Input: dimensioned drawing with shaded views. Units: mm. Origin: part minimum x, y, z. A direction names the side the tool comes from. Round coordinates to 2 decimals unless told otherwise and drop trailing zeros. Loops run counter-clockwise (first coordinate to the right, second up) from the corner with the lowest first, then second, coordinate; pieces in that order, holes last.
Item 1: Pull-direction query (Z, two-part tool) for the marked faces 3, 4 and 5; classes: released by +Z, released by -Z, zero draft, split by the parting line, or undercut.
Item 2: First-contact query: P1, Ø1, axis at y = 2.5, z = 9.5, coming from the -X side; P2, Ø5, axis at x = 5.75, z = 6.75, coming from the -Y side. Flat tips, straight axial feed; report the tip coordinate or a pass-through.
Item 3: Section query B-B on z = 6.75. Return loops of the section in (x, y).
Item 4: Ray query, L1, parallel to X at y = 5.65, z = 6.75; L2, parallel to Z at x = 5.75, y = 5.3; L3, parallel to X at y = 1, z = 7. Return the intervals inside material, ascending.
Item 5: Access query for the marked faces 1 and 2. Directions: +Z, -Z, +X, -X, +Y, -Y. A direction counts if a zero-diameter tool reaches every point of the face in a straight line with its end or side. Return the directions, or none.
Item 6: Section query A-A on x = 5.75. Return loops of the section in (y, z).
Item 7: Section query D-D on z = 4. Return loops of the section in (x, y), then the cut area to 4 significant figures.
Item 8: Section query C-C on y = 6. Return loops of the section in (x, z), then the cut area to 3 significant figures.
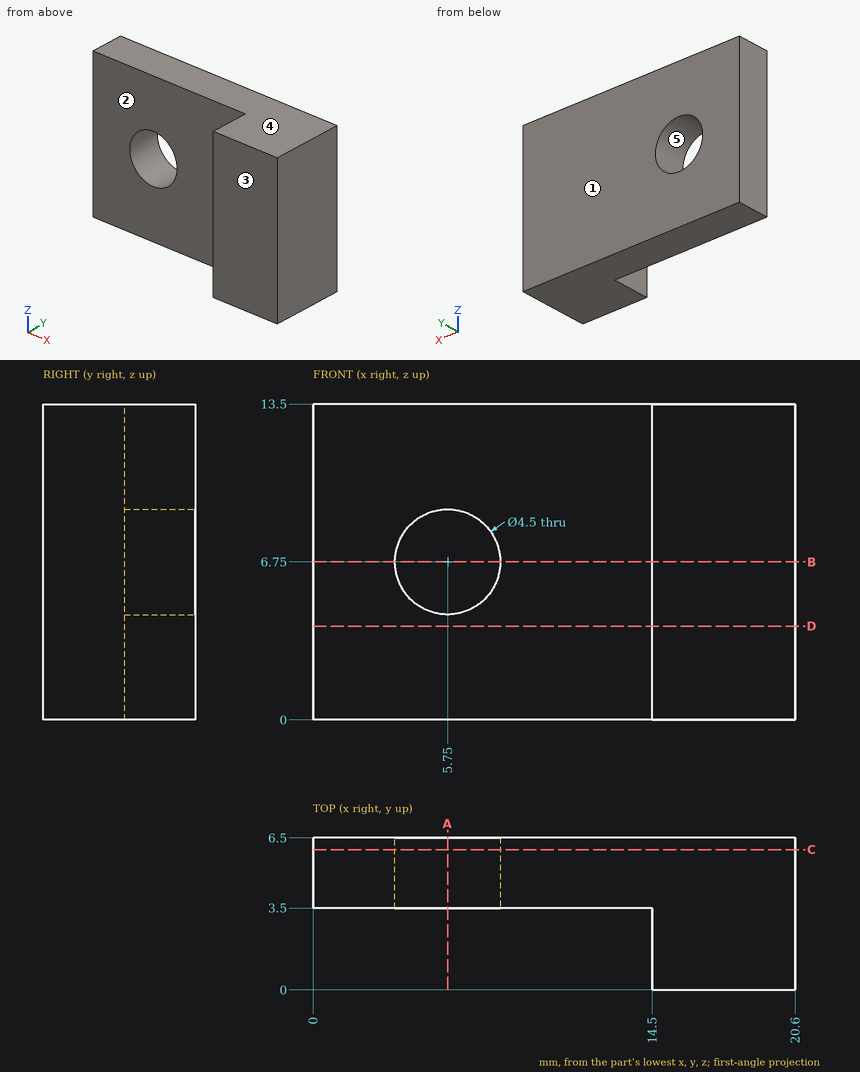
Data:
1. face 3: zero draft
1. face 4: released by +Z
1. face 5: undercut
2. P1: stops at x = 14.5
2. P2: stops at y = 3.5
3. outline: (0, 3.5) - (3.5, 3.5) - (3.5, 6.5) - (0, 6.5) - close; (8, 3.5) - (14.5, 3.5) - (14.5, 0) - (20.6, 0) - (20.6, 6.5) - (8, 6.5) - close
4. L1: x = 0 to 3.5, 8 to 20.6
4. L2: z = 0 to 4.5, 9 to 13.5
4. L3: x = 14.5 to 20.6
5. face 1: +Z, -Z, +X, -X, +Y
5. face 2: +Z, -Z, -X, -Y
6. outline: (3.5, 0) - (6.5, 0) - (6.5, 4.5) - (3.5, 4.5) - close; (3.5, 9) - (6.5, 9) - (6.5, 13.5) - (3.5, 13.5) - close
7. outline: (0, 3.5) - (14.5, 3.5) - (14.5, 0) - (20.6, 0) - (20.6, 6.5) - (0, 6.5) - close
7. area: 83.15 mm2
8. outline: (0, 0) - (20.6, 0) - (20.6, 13.5) - (0, 13.5) - close; hole circle Ø4.5 at (5.75, 6.75)
8. area: 262 mm2
